Read the model definition and answer for the solid it produces. Units are mm, in the model's axes. Face numbers are marked on the shaded views. Give positions to 0.01 mm unless a question says otherwise; leave off trailing zeros. Write each loop counter-clockwise with the first axis right and the second up, starting at its lowest first coordinate (ties: lowest second). Pieces come first, ordered by that corner, then holes.
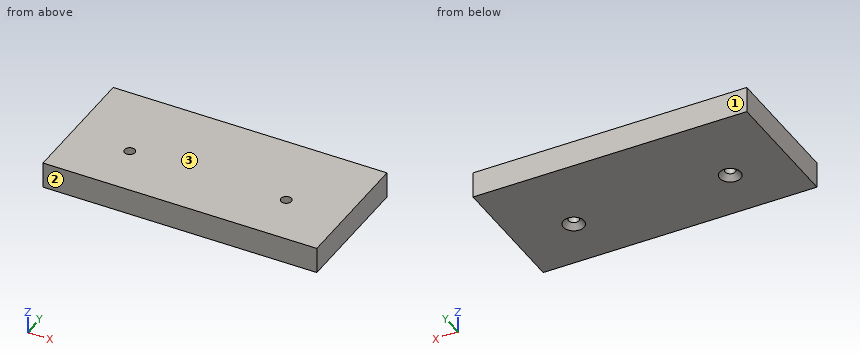
```python
from build123d import *

# Parameters (mm, degrees)
F0_W     = 105
F0_H     = 50
F1_DEPTH = 10
F3_DEPTH = 10.001
F4_SIZE  = 2


with BuildPart() as f1:
    # F0 (on Top) → F1 (new body)
    with BuildSketch(Plane.XY):
        Rectangle(F0_W, F0_H)
    extrude(amount=F1_DEPTH)

    # F2 (on face) → F3 (cut, through all)
    with BuildSketch(Plane.XY.offset(10)):
        with BuildLine():
            ThreePointArc((-28, -5), (-30, -3), (-32, -5))
            Line((-32, -5), (-28, -5))
        make_face()
        with BuildLine():
            Line((-28, -5), (-32, -5))
            ThreePointArc((-32, -5), (-30, -7), (-28, -5))
        make_face()
        with BuildLine():
            ThreePointArc((32, -5), (30, -3), (28, -5))
            Line((28, -5), (32, -5))
        make_face()
        with BuildLine():
            Line((32, -5), (28, -5))
            ThreePointArc((28, -5), (30, -7), (32, -5))
        make_face()
    extrude(amount=-F3_DEPTH, mode=Mode.SUBTRACT)

    # F4
    f4_edges = [f1.edges().sort_by_distance(p)[0] for p in [
        (32, -5, 0),
        (-28, -5, 0),
    ]]
    chamfer(f4_edges, length=F4_SIZE)


solid = f1.part
```
Item 1: This flat-tipped pin is pushed along its axis until it touches: pin 1 Ø4.5 at (x, y) = (30, -5) entering from -Z. Where does it stop, or does it pass through?
Result set:
pin 1: stops at z = 1.75
Item 2: Determine the mould class of the marked faces 1, 2 and 3 for opening direction Y: pulls with the +Y half, pulls with the -Y half, needs draft (parallel to the pull), parting line crosses it, or undercut.
Result set:
face 1: pulls with the +Y half
face 2: pulls with the -Y half
face 3: needs draft
Item 3: Section A-A (x = 30) is taken. Write down the section's boundary in (y, z), and give its area (3 significant figures).
Result set:
outline: (-25, 0) - (-9, 0) - (-7, 2) - (-7, 10) - (-25, 10) - close; (-3, 2) - (-1, 0) - (25, 0) - (25, 10) - (-3, 10) - close
area: 456 mm2
Item 4: Find the intervals of material crossed by line 1 along X through (y, z) = (-5, 6.25); line 2 along Y through (x, z) = (-30, 7.75); line 3 along Z through (x, y) = (-29, -8.5), in increasing order.
Result set:
line 1: x = -52.5 to -32, -28 to 28, 32 to 52.5
line 2: y = -25 to -7, -3 to 25
line 3: z = 0.36 to 10
Item 5: Section B-B (y = -5) is taken. Write down the section's boundary in (x, z).
Result set:
outline: (-52.5, 0) - (-34, 0) - (-32, 2) - (-32, 10) - (-52.5, 10) - close; (-28, 2) - (-26, 0) - (26, 0) - (28, 2) - (28, 10) - (-28, 10) - close; (32, 2) - (34, 0) - (52.5, 0) - (52.5, 10) - (32, 10) - close
